Model file for the job. Use its own axes, mm. Give positions to 0.01 mm unless a question says otherwise; leave off trailing zeros. Loops run counter-clockwise (first coordinate to the right, second up) from the corner with the lowest first, then second, coordinate; pieces in that order, holes last. Notation, with made-up numbers: M -19,59 L -13,59 A28 ccw -13,84 Z; hole C 31,49 d9. An arc over 180 degrees is marked long. Answer in a Markdown table with one row per item.
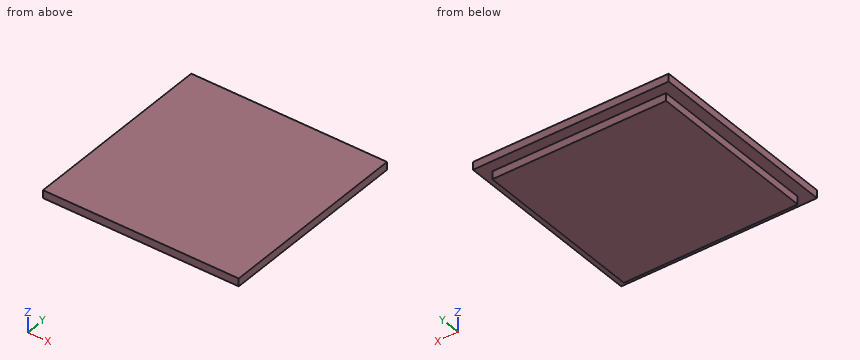
```python
from build123d import *

# Parameters (mm, degrees)
F0_W     = 44.4
F0_H     = 44.4
F1_DEPTH = 2
F0_W_2   = 50
F0_H_2   = 50
F2_DEPTH = 2


with BuildPart() as f1:
    # F0 (on Top) → F1 (new body)
    with BuildSketch(Plane.XY):
        Rectangle(F0_W, F0_H)
    extrude(amount=-F1_DEPTH)

    # F0 (on Top) → F2 (join)
    with BuildSketch(Plane.XY):
        Rectangle(F0_W_2, F0_H_2)
        Rectangle(F0_W, F0_H, mode=Mode.SUBTRACT)
        Rectangle(F0_W, F0_H)
    extrude(amount=F2_DEPTH)


solid = f1.part
```
(1) Flat gauge pins, fed straight in: P1, Ø1.6, axis at y = -3.5, z = -1.5, coming from the -X side; P2, Ø1.6, axis at x = -5.5, z = -1, coming from the +Y side; P3, Ø1.5, axis at x = 9.5, z = -1, coming from the -Y side. Where does each tip first touch, or does it go through?
Established:
| item | result |
|---|---|
| P1 | stops at x = -22.2 |
| P2 | stops at y = 22.2 |
| P3 | stops at y = -22.2 |
(2) Saw through at C-C, the plane z = -1.05. Give the cut face in (x, y).
Established:
| item | result |
|---|---|
| outline | M -22.2,-22.2 L 22.2,-22.2 L 22.2,22.2 L -22.2,22.2 Z |
(3) Wall check: L1, parallel to X at y = -3.5, z = -1.8; L2, parallel to Z at x = -22.5, y = -6. Give the ranges that are in metal, low to high.
Established:
| item | result |
|---|---|
| L1 | x = -22.2 to 22.2 |
| L2 | z = 0 to 2 |
(4) Saw through at A-A, the plane x = -20. Give the cut face in (y, z).
Established:
| item | result |
|---|---|
| outline | M -25,0 L -22.2,0 L -22.2,-2 L 22.2,-2 L 22.2,0 L 25,0 L 25,2 L -25,2 Z |
